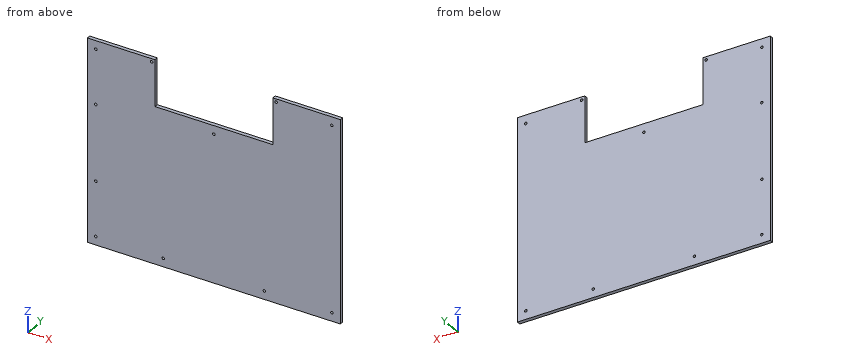
from build123d import *

# Parameters (mm, degrees)
BOSS_EXTRUDE1_DEPTH   = 5.588
F_6_CLEARANCE_HOLE1_D = 3.7973


with BuildPart() as part:
    # Sketch1 → Boss-Extrude1 (new body)
    with BuildSketch(Plane(origin=(0, 0, 0), x_dir=(1, 0, 0), z_dir=(0, 1, 0))):
        Polygon((-190.5, -152.4), (-88.9, -152.4), (-88.9, -82.55), (88.9, -82.55), (88.9, -152.4), (190.5, -152.4), (190.5, 152.4), (-190.5, 152.4), align=None)
    extrude(amount=BOSS_EXTRUDE1_DEPTH)

    # #6 Clearance Hole1 (through all)
    with Locations(Plane(origin=(-76.2, 5.588, -139.7), x_dir=(0, 0, 1), z_dir=(0, 1, 0))):
        with Locations((0, 0), (0, 152.4), (209.55, 76.2), (287.3248, -17.4752), (279.4, -101.6), (0, -101.6), (0, 254), (279.4, 254), (287.3248, 169.8752), (82.55, -101.6), (196.85, -101.6)):
            Hole(F_6_CLEARANCE_HOLE1_D / 2)


solid = part.part
CAD build for the part. Positions are in the model's coordinates, mm. Give positions to 0.01 mm unless a question says otherwise; leave off trailing zeros. Order: outer loops, then holes, each group sorted by start corner. A loop starts at its lowest first (then second) coordinate and runs counter-clockwise, first axis right, second up. Notation, with made-up numbers: (-3.75, 79) - (10.25, 79) arc R30 cw to (10.25, 101) - close; hole circle Ø6 at (50.5, 49.5). An arc over 180 degrees is marked (long way). Answer in a Markdown table with one row per item.
1. Saw through at B-B, the plane y = 2.35. Count the separate pieces of the cut face and the enclosed holes in it, plus the area to 3 significant figures.
Data:
| item | result |
|---|---|
| separate pieces | 1 |
| enclosed holes | 11 |
| area | 104,000 mm² |
2. Saw through at C-C, the plane x = 50. Give the cut face in (y, z).
Data:
| item | result |
|---|---|
| outline | (0, -152.4) - (5.59, -152.4) - (5.59, 82.55) - (0, 82.55) - close |
3. Saw through at A-A, the plane z = 92.5. Give the cut face in (x, y).
Data:
| item | result |
|---|---|
| outline | (-190.5, 0) - (-88.9, 0) - (-88.9, 5.59) - (-190.5, 5.59) - close; (88.9, 0) - (190.5, 0) - (190.5, 5.59) - (88.9, 5.59) - close |
4. Flat gauge pin, fed straight in: pin 1 (1.7 mm diameter, centred on x = 41, y = 1.5, fed in from +Z). Where does the tip first touch, or does it go through?
Data:
| item | result |
|---|---|
| pin 1 | stops at z = 82.55 |
5. Probe probe 1 along X at (y, z) = (2.7, -139.7); probe 2 along X at (y, z) = (4.7, 123.5); probe 3 along Z at (x, y) = (-0.5, 2.4). List the from-to ranges inside material, lowest first. Write a range as [from, to].
Data:
| item | result |
|---|---|
| probe 1 | x = [-190.5, -179.7], [-175.9, -78.1], [-74.3, 74.3], [78.1, 175.9], [179.7, 190.5] |
| probe 2 | x = [-190.5, -88.9], [88.9, 190.5] |
| probe 3 | z = [-152.4, 68.02], [71.68, 82.55] |
